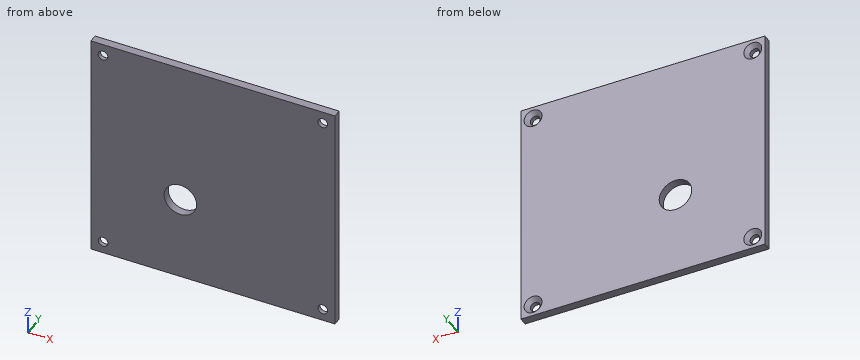
```python
from build123d import *

# Parameters (mm, degrees)
SKETCH1_W                                    = 60
SKETCH1_H                                    = 57
BOSS_EXTRUDE1_DEPTH                          = 2
CSK_FOR_M2_COUNTERSUNK_FLAT_HEAD_SCR_2_COUNT = 2
CSK_FOR_M2_COUNTERSUNK_FLAT_HEAD_SCR_2_PITCH = 54
CSK_FOR_M2_COUNTERSUNK_FLAT_HEAD_SCR_3_COUNT = 2
CSK_FOR_M2_COUNTERSUNK_FLAT_HEAD_SCR_3_PITCH = 74.276510419
CSK_FOR_M2_COUNTERSUNK_FLAT_HEAD_SCR_4_COUNT = 2
CSK_FOR_M2_COUNTERSUNK_FLAT_HEAD_SCR_4_PITCH = 51
SKETCH4_R                                    = 4
CUT_EXTRUDE1_DEPTH                           = 2


with BuildPart() as part:
    # Sketch1 → Boss-Extrude1 (new body)
    with BuildSketch(Plane(origin=(0, 0, 0), x_dir=(1, 0, 0), z_dir=(0, 1, 0))):
        Rectangle(SKETCH1_W, SKETCH1_H)
    extrude(amount=BOSS_EXTRUDE1_DEPTH)

    # Sketch3 → CSK for M2 Countersunk Flat Head Screw1 (revolve, cut)
    with BuildSketch(Plane(origin=(-27, 2, -25.5), x_dir=(0, 0, 1), z_dir=(1, 0, 0))):
        Polygon((0, 0), (0, 2), (1.2, 2), (1.2, 1), (2.2, 0), align=None)
    csk_for_m2_countersunk_flat_head_screw1 = revolve(axis=Axis((-27, 8.35, -25.5), (0, -1, 0)), mode=Mode.SUBTRACT)

    # CSK for M2 Countersunk Flat Head Scr 2: CSK for M2 Countersunk Flat Head Screw1 ×2
    with Locations(*[(i * CSK_FOR_M2_COUNTERSUNK_FLAT_HEAD_SCR_2_PITCH, 0, 0) for i in range(1, CSK_FOR_M2_COUNTERSUNK_FLAT_HEAD_SCR_2_COUNT)]):
        add(csk_for_m2_countersunk_flat_head_screw1, mode=Mode.SUBTRACT)

    # CSK for M2 Countersunk Flat Head Scr 3: CSK for M2 Countersunk Flat Head Screw1 ×2
    with Locations(*[Vector(0.7270131525498175, 0, 0.6866235329637166) * (i * CSK_FOR_M2_COUNTERSUNK_FLAT_HEAD_SCR_3_PITCH) for i in range(1, CSK_FOR_M2_COUNTERSUNK_FLAT_HEAD_SCR_3_COUNT)]):
        add(csk_for_m2_countersunk_flat_head_screw1, mode=Mode.SUBTRACT)

    # CSK for M2 Countersunk Flat Head Scr 4: CSK for M2 Countersunk Flat Head Screw1 ×2
    with Locations(*[(0, 0, i * CSK_FOR_M2_COUNTERSUNK_FLAT_HEAD_SCR_4_PITCH) for i in range(1, CSK_FOR_M2_COUNTERSUNK_FLAT_HEAD_SCR_4_COUNT)]):
        add(csk_for_m2_countersunk_flat_head_screw1, mode=Mode.SUBTRACT)

    # Sketch4 → Cut-Extrude1 (cut)
    with BuildSketch(Plane(origin=(0, 2, 0), x_dir=(1, 0, 0), z_dir=(0, 1, 0))):
        with Locations(Location((-8, 7.5, 0), (0, 0, 270))):
            Circle(SKETCH4_R)
    extrude(amount=-CUT_EXTRUDE1_DEPTH, mode=Mode.SUBTRACT)


solid = part.part
```
Model file for the job. Use its own axes, mm. Coordinates: 2 decimals unless noted, no trailing zeros. Write each loop counter-clockwise with the first axis right and the second up, starting at its lowest first coordinate (ties: lowest second). Pieces come first, ordered by that corner, then holes. Notation, with made-up numbers: (78, 63.5) - (96, 63.5) arc R20 ccw to (96, 78.5) - close; hole circle Ø1 at (-15.75, -14.75). An arc over 180 degrees is marked (long way). One line per item, written item: value. Start each with the question number.
1. Flat gauge pins, fed straight in: pin 1 (13 mm diameter, centred on x = -8, z = -7.5, fed in from +Y); pin 2 (3 mm diameter, centred on x = -27, z = 25.5, fed in from +Y); pin 3 (2 mm diameter, centred on x = 27, z = 25.5, fed in from +Y). Where does each tip first touch, or does it go through?
2. Slice it at B-B (x = 27). Write the cut outline in (y, z), plus the area to 3 significant figures.
3. Probe line 1 (X direction, y = 0.7, z = -25.5); line 2 (X direction, y = 0.55, z = -7.5); line 3 (Z direction, x = -7, y = 0.55). List the from-to ranges inside material, lowest first. Write a range as from..to.
4. Slice it at C-C (y = 1.35). Write the cut outline in (x, z).
5. Slice it at D-D (z = -7.5). Write the cut outline in (x, y), plus the area to 3 significant figures.
6. Slice it at A-A (z = -25.5). Write the cut outline in (x, y).
Answers below:
1. pin 1: stops at y = 2
1. pin 2: stops at y = 1.3
1. pin 3: passes through
2. outline: (0, -28.5) - (2, -28.5) - (2, -27.7) - (1, -26.7) - (0, -26.7) - close; (0, -24.3) - (1, -24.3) - (2, -23.3) - (2, 23.3) - (1, 24.3) - (0, 24.3) - close; (0, 26.7) - (1, 26.7) - (2, 27.7) - (2, 28.5) - (0, 28.5) - close
2. area: 102 mm^2
3. line 1: x = -30..-28.2, -25.8..25.8, 28.2..30
3. line 2: x = -30..-12, -4..30
3. line 3: z = -28.5..-11.37, -3.63..28.5
4. outline: (-30, -28.5) - (30, -28.5) - (30, 28.5) - (-30, 28.5) - close; hole circle Ø3.1 at (-27, -25.5); hole circle Ø3.1 at (-27, 25.5); hole circle Ø8 at (-8, -7.5); hole circle Ø3.1 at (27, -25.5); hole circle Ø3.1 at (27, 25.5)
5. outline: (-30, 0) - (-12, 0) - (-12, 2) - (-30, 2) - close; (-4, 0) - (30, 0) - (30, 2) - (-4, 2) - close
5. area: 104 mm^2
6. outline: (-30, 0) - (-28.2, 0) - (-28.2, 1) - (-29.2, 2) - (-30, 2) - close; (-25.8, 0) - (25.8, 0) - (25.8, 1) - (24.8, 2) - (-24.8, 2) - (-25.8, 1) - close; (28.2, 0) - (30, 0) - (30, 2) - (29.2, 2) - (28.2, 1) - close
